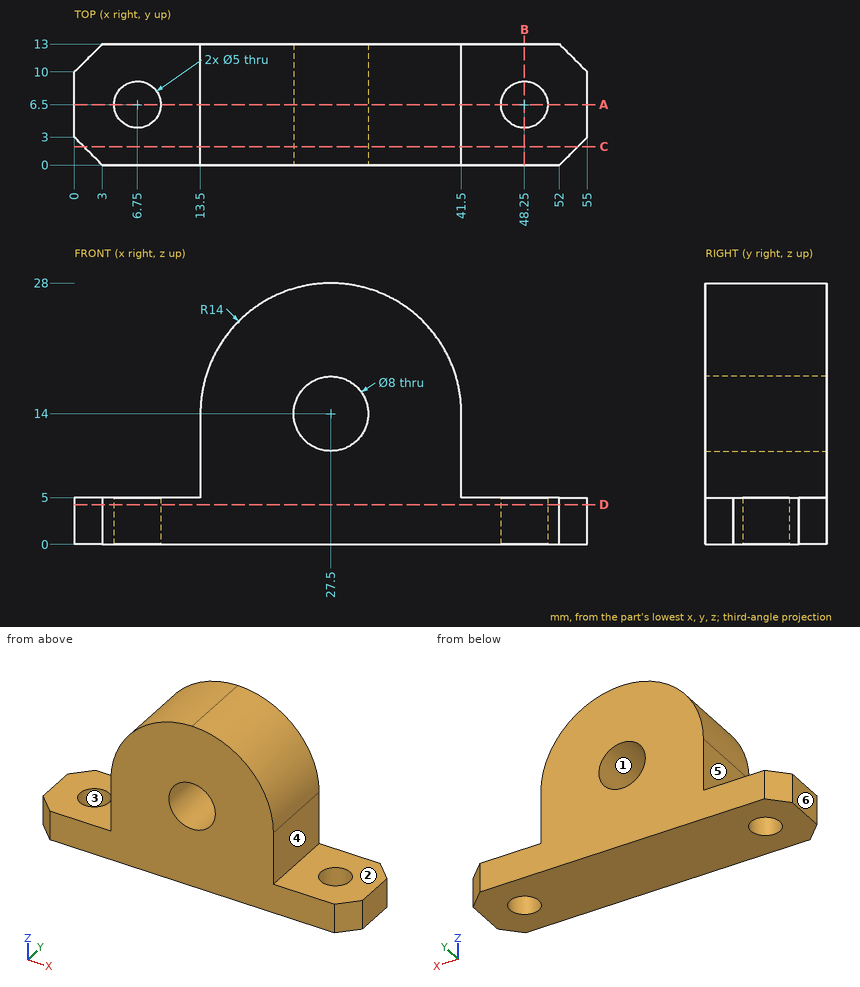
Could you check a few things on this drawing? It's one solid part, dimensions in mm from its lowest x, y, z. A direction names the side the tool comes from. Coordinates: 2 decimals unless noted, no trailing zeros. Order: outer loops, then holes, each group sorted by start corner. A loop starts at its lowest first (then second) coordinate and runs counter-clockwise, first axis right, second up. Notation, with made-up numbers: M 57,70.25 L 93,70.25 A25 cw 93,88.25 Z; hole C -29.5,-7 d1. An arc over 180 degrees is marked long. Use a Markdown table: item, result. Add a question column.
Q1. If I drill on L1, parallel to X at y = 7, z = 14; L2, parallel to Y at x = 48.25, z = 3.65; L3, parallel to Z at x = 3.5, y = 1.5, over which ranges is the centre line in solid material (lowest first)?
Q2. I want a section at D-D on z = 4.25. List the corners of the cut face in (x, y) for me.
Q3. I want a section at C-C on y = 2. List the corners of the cut face in (x, z) for me, then the cut area to 3 significant figures.
Q4. I'm going to push flat-ended pins straight in: pin 1 (7 mm diameter, centred on x = 27.5, z = 14, fed in from +Y); pin 2 (2.5 mm diameter, centred on y = 5.5, z = 11, fed in from +X); pin 3 (2.5 mm diameter, centred on y = 8.5, z = 10.5, fed in from -X); pin 4 (6.5 mm diameter, centred on x = 4, y = 9.5, fed in from +Z). Where does each tip first touch, or does it pass through?
Q5. I want a section at A-A on y = 6.5. List the corners of the cut face in (x, z) for me, then the cut area to 3 significant figures.
Q6. We'd pull the mould along Z, two halves only. Please class the marked faces 1, 2 and 3: pulls with the +Z half, pulls with the -Z half, needs draft (parallel to the pull), parting line crosses it, or undercut.
Q7. I want a section at B-B on x = 48.25. List the corners of the cut face in (y, z) for me.
Q8. Which directions (+Z, -Z, +X, -X, +Y, -Y) give clear straight access to the entire face, cutting with the end or side of a thin tool? Please do the marked faces 4, 5 and 6.
Checked values:
| question | item | result |
|---|---|---|
| 1 | L1 | 13.5 to 23.5, 31.5 to 41.5 |
| 1 | L2 | 0 to 4, 9 to 13 |
| 1 | L3 | 0 to 5 |
| 2 | outline | M 0,3 L 3,0 L 52,0 L 55,3 L 55,10 L 52,13 L 3,13 L 0,10 Z; hole C 6.75,6.5 d5; hole C 48.25,6.5 d5 |
| 3 | outline | M 1,0 L 54,0 L 54,5 L 41.5,5 L 41.5,14 A14 ccw 13.5,14 L 13.5,5 L 1,5 Z; hole C 27.5,14 d8 |
| 3 | area | 775 mm² |
| 4 | pin 1 | through |
| 4 | pin 2 | x = 41.5 |
| 4 | pin 3 | x = 13.5 |
| 4 | pin 4 | z = 5 |
| 5 | outline | M 0,0 L 4.25,0 L 4.25,5 L 0,5 Z; M 9.25,0 L 45.75,0 L 45.75,5 L 41.5,5 L 41.5,14 A14 ccw 13.5,14 L 13.5,5 L 9.25,5 Z; M 50.75,0 L 55,0 L 55,5 L 50.75,5 Z; hole C 27.5,14 d8 |
| 5 | area | 735 mm² |
| 6 | face 1 | undercut |
| 6 | face 2 | pulls with the +Z half |
| 6 | face 3 | needs draft |
| 7 | outline | M 0,0 L 4,0 L 4,5 L 0,5 Z; M 9,0 L 13,0 L 13,5 L 9,5 Z |
| 8 | face 4 | +Z, +X, +Y, -Y |
| 8 | face 5 | +Z, -X, +Y, -Y |
| 8 | face 6 | +Z, -Z, -X, +Y, -Y |
